from build123d import *

# Parameters (mm, degrees)
F1_DEPTH = 873.125
F2_W     = 304.8
F2_H     = 171.45
F2_R     = 17.4625
F2_W_2   = 234.95
F3_DEPTH = 25.4
F4_W     = 12.7
F4_H     = 762
F5_DEPTH = 352.425


with BuildPart() as f1:
    # F0 (on Right) → F1 (new body, symmetric)
    with BuildSketch(Plane.YZ):
        with BuildLine():
            ThreePointArc((381, 31.75), (390.29936, 9.29936), (412.75, 0))
            Line((412.75, 0), (520.7, 0))
            Line((520.7, 0), (520.7, 12.7))
            Line((520.7, 12.7), (412.75, 12.7))
            ThreePointArc((412.75, 12.7), (399.279616, 18.279616), (393.7, 31.75))
            Line((393.7, 31.75), (393.7, 333.375))
            ThreePointArc((393.7, 333.375), (384.40064, 355.82564), (361.95, 365.125))
            Line((361.95, 365.125), (0, 365.125))
            Line((0, 365.125), (-361.95, 365.125))
            ThreePointArc((-361.95, 365.125), (-384.40064, 355.82564), (-393.7, 333.375))
            Line((-393.7, 333.375), (-393.7, 31.75))
            ThreePointArc((-393.7, 31.75), (-399.279616, 18.279616), (-412.75, 12.7))
            Line((-412.75, 12.7), (-520.7, 12.7))
            Line((-520.7, 12.7), (-520.7, 0))
            Line((-520.7, 0), (-412.75, 0))
            ThreePointArc((-412.75, 0), (-390.29936, 9.29936), (-381, 31.75))
            Line((-381, 31.75), (-381, 333.375))
            ThreePointArc((-381, 333.375), (-375.420384, 346.845384), (-361.95, 352.425))
            Line((-361.95, 352.425), (0, 352.425))
            Line((0, 352.425), (361.95, 352.425))
            ThreePointArc((361.95, 352.425), (375.420384, 346.845384), (381, 333.375))
            Line((381, 333.375), (381, 31.75))
        make_face()
    extrude(amount=F1_DEPTH, both=True)

    # F2 (on face) → F3 (join)
    with BuildSketch(Plane.XY.offset(365.125)):
        with Locations((238.125, 269.875)):
            Rectangle(F2_W, F2_H)
        with Locations((282.575, 285.75)):
            Circle(F2_R, mode=Mode.SUBTRACT)
        with Locations((-431.8, 269.875)):
            Rectangle(F2_W_2, F2_H)
        with Locations((-441.325, 285.75)):
            Circle(F2_R, mode=Mode.SUBTRACT)
        with Locations((238.125, -269.875)):
            Rectangle(F2_W, F2_H)
        with Locations((282.575, -285.75)):
            Circle(F2_R, mode=Mode.SUBTRACT)
        with Locations((-431.8, -269.875)):
            Rectangle(F2_W_2, F2_H)
        with Locations((-441.325, -285.75)):
            Circle(F2_R, mode=Mode.SUBTRACT)
    extrude(amount=F3_DEPTH)

    # F4 (on face) → F5 (join, through all)
    with BuildSketch(Plane(origin=(0, 0, 352.425), x_dir=(1, 0, 0), z_dir=(0, 0, -1))):
        with Locations((688.975, 0)):
            Rectangle(F4_W, F4_H)
    extrude(amount=F5_DEPTH)


solid = f1.part
Input: part model. Units: mm. Frame: model coordinates. A direction names the side the tool comes from. Coordinates: 2 decimals unless noted, no trailing zeros. Loops run counter-clockwise (first coordinate to the right, second up) from the corner with the lowest first, then second, coordinate; pieces in that order, holes last. Notation, with made-up numbers: (-38.75, 54.5) -> (-20.75, 54.5) arc R36 cw to (-20.75, 90.5) -> close; hole circle Ø2 at (54.25, 17.25). An arc over 180 degrees is marked (long way). One line per item, written item: value.
(1) Draft query along X for faces 5 (the face through (873.125, -2, 359)), 6 (the face through (283, -286, 365.125)), 7 (the face through (-433, -269, 390.525)). Return one class per face: pulls with the +X half, pulls with the -X half, needs draft (parallel to the pull), parting line crosses it, or undercut.
Answer below:
face 5: pulls with the +X half
face 6: undercut
face 7: needs draft
(2) Cut plane B-B (x = -761.5). Output: boundary loops of the cut face in (y, z) (3 decimals), then the cut area to 3 significant figures.
Answer below:
outline: (-520.7, 0) -> (-412.75, 0) arc R31.75 ccw to (-381, 31.75) -> (-381, 333.375) arc R19.05 cw to (-361.95, 352.425) -> (361.95, 352.425) arc R19.05 cw to (381, 333.375) -> (381, 31.75) arc R31.75 ccw to (412.75, 0) -> (520.7, 0) -> (520.7, 12.7) -> (412.75, 12.7) arc R19.05 cw to (393.7, 31.75) -> (393.7, 333.375) arc R31.75 ccw to (361.95, 365.125) -> (-361.95, 365.125) arc R31.75 ccw to (-393.7, 333.375) -> (-393.7, 31.75) arc R19.05 cw to (-412.75, 12.7) -> (-520.7, 12.7) -> close
area: 21,600 mm2
(3) Cut plane A-A (y = -18). Output: boundary loops of the cut face in (x, z) (3 decimals).
Answer below:
outline: (-873.125, 352.425) -> (682.625, 352.425) -> (682.625, 0) -> (695.325, 0) -> (695.325, 352.425) -> (873.125, 352.425) -> (873.125, 365.125) -> (-873.125, 365.125) -> close
(4) Ray query, line 1 along X through (y, z) = (-285, 375) (3 decimals); line 2 along Y through (x, z) = (-575.5, 300); line 3 along Y through (x, z) = (-669.5, 29). Return the intervals inside material, ascending.
Answer below:
line 1: x = -549.275 to -458.771, -423.879 to -314.325, 85.725 to 265.129, 300.021 to 390.525
line 2: y = -393.7 to -381, 381 to 393.7
line 3: y = -393.9 to -381.12, 381.12 to 393.9
(5) Cut plane C-C (z = 161.5). Output: boundary loops of the cut face in (x, y) (3 decimals), then the cut area to 3 significant figures.
Answer below:
outline: (-873.125, -393.7) -> (873.125, -393.7) -> (873.125, -381) -> (695.325, -381) -> (695.325, 381) -> (873.125, 381) -> (873.125, 393.7) -> (-873.125, 393.7) -> (-873.125, 381) -> (682.625, 381) -> (682.625, -381) -> (-873.125, -381) -> close
area: 54,000 mm2
(6) Set-up query: faces 1 (the face through (12, 467, 12.7)), 2 (the face through (785, -381, 180)), 3 (the face through (-458.77, 286.52, 377.65)), 4 (the face through (-84, -5, 352.425)). Return all of +Z, -Z, +X, -X, +Y, -Y with unobstructed straight access to the full face (end or side cutting, diameter ignored); none if empty.
Answer below:
face 1: +Z, +X, -X, +Y
face 2: -Z, +X
face 3: +Z
face 4: -Z, -X
(7) Pin query (flat end, axial travel): pin 1 Ø7.5 at (y, z) = (-242.5, 384) entering from +X (3 decimals); pin 2 Ø6 at (x, z) = (598, 230) entering from -Y; pin 3 Ø12.5 at (x, z) = (229.5, 375) entering from +Y. Return the tip coordinate at first contact, or that it passes through.
Answer below:
pin 1: stops at x = 390.525
pin 2: stops at y = -393.7
pin 3: stops at y = 355.6
(8) Cut plane D-D (x = -491). Output: boundary loops of the cut face in (y, z) (3 decimals), then the cut area to 3 significant figures.
Answer below:
outline: (-520.7, 0) -> (-412.75, 0) arc R31.75 ccw to (-381, 31.75) -> (-381, 333.375) arc R19.05 cw to (-361.95, 352.425) -> (361.95, 352.425) arc R19.05 cw to (381, 333.375) -> (381, 31.75) arc R31.75 ccw to (412.75, 0) -> (520.7, 0) -> (520.7, 12.7) -> (412.75, 12.7) arc R19.05 cw to (393.7, 31.75) -> (393.7, 333.375) arc R31.75 ccw to (361.95, 365.125) -> (355.6, 365.125) -> (355.6, 390.525) -> (184.15, 390.525) -> (184.15, 365.125) -> (-184.15, 365.125) -> (-184.15, 390.525) -> (-355.6, 390.525) -> (-355.6, 365.125) -> (-361.95, 365.125) arc R31.75 ccw to (-393.7, 333.375) -> (-393.7, 31.75) arc R19.05 cw to (-412.75, 12.7) -> (-520.7, 12.7) -> close
area: 30,300 mm2
